Model file for the job. Use its own axes, mm. Round coordinates to 2 decimals unless told otherwise and drop trailing zeros. Order: outer loops, then holes, each group sorted by start corner. A loop starts at its lowest first (then second) coordinate and runs counter-clockwise, first axis right, second up. Notation, with made-up numbers: (-17, -2) - (-9, -2) arc R27 ccw to (-9, 20) - close; hole circle Ø7 at (73, 66). An arc over 180 degrees is marked (long way). Answer as CSV lines item,"result". Start each with the question number.
1. Band-saw the part on B-B on z = -216. List the corners of the cut face in (x, y).
2. Wall check: line 1 along X through (y, z) = (463.25, -150.5); line 2 along Z through (x, y) = (-190.5, 450.5); line 3 along Z through (x, y) = (-132, 465.75). Give the ranges that are in metal, low to high. Write a range as [from, to].
3. Pin check, flat tip, straight feed: pin 1 Ø3 at (x, y) = (-106, 451.5) entering from -Z. Stop position of the tip, or through.
4. Band-saw the part on A-A on x = -104. List the corners of the cut face in (y, z).
```python
from build123d import *

# Parameters (mm, degrees)
BOSS_EXTRUDE1_START = 116
SKETCH1_W           = 160
SKETCH1_H           = 130
SKETCH1_W_2         = 154
SKETCH1_H_2         = 124
BOSS_EXTRUDE1_DEPTH = 2


with BuildPart() as part:
    # Sketch1 → Boss-Extrude1 (new body)
    with BuildSketch(Plane(origin=(0, 358.879876801, -41.422455829), x_dir=(1, 0, 0), z_dir=(-6.837425950214788e-15, 0.9934047622419533, -0.1146602736566085)).offset(BOSS_EXTRUDE1_START)):
        with Locations((-135, 150.244347434)):
            Rectangle(SKETCH1_W, SKETCH1_H)
        with Locations((-135, 150.244347434)):
            Rectangle(SKETCH1_W_2, SKETCH1_H_2, mode=Mode.SUBTRACT)
    extrude(amount=BOSS_EXTRUDE1_DEPTH)


solid = part.part
```
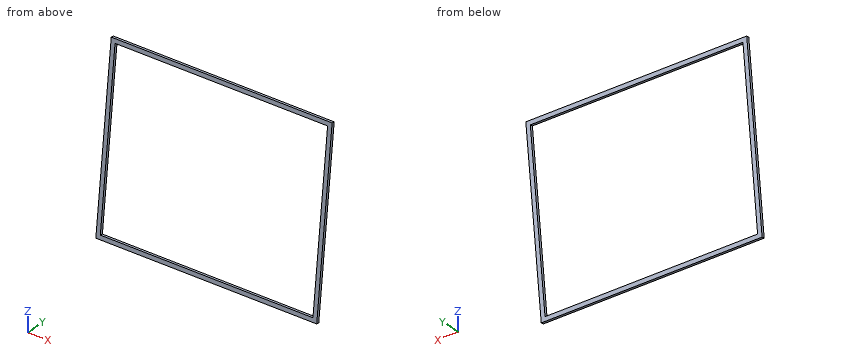
Reply:
1,outline,"(-215, 455.5) - (-212, 455.5) - (-212, 457.51) - (-215, 457.51) - close; (-58, 455.5) - (-55, 455.5) - (-55, 457.51) - (-58, 457.51) - close"
2,line 1,"x = [-215, -212], [-58, -55]"
2,line 2,"z = [-268.67, -265.65]"
2,line 3,"z = [-142.59, -139.57]"
3,pin 1,"stops at z = -268.78"
4,outline,"(449.43, -268.55) - (451.42, -268.78) - (451.77, -265.8) - (449.78, -265.57) - close; (464, -142.39) - (465.98, -142.61) - (466.33, -139.63) - (464.34, -139.41) - close"
